Part model, mm, in its own coordinate system. Round coordinates to 2 decimals unless told otherwise and drop trailing zeros. Write each loop counter-clockwise with the first axis right and the second up, starting at its lowest first coordinate (ties: lowest second). Pieces come first, ordered by that corner, then holes. Notation, with made-up numbers: M 2,-32.5 L 9,-32.5 A6 ccw 9,-26.5 Z; hole C 3.25,-0.5 d6. An arc over 180 degrees is marked long. Use one line per item in the form item = value. Start each with the question number.
Item 1: Probe L1, parallel to Z at x = 0, y = -6; L2, parallel to Y at x = -2.5, z = 0.25; L3, parallel to X at y = -9, z = 0.25. List the from-to ranges inside material, lowest first.
Item 2: Cut at C-C, the plane z = -2.75. Give the cut face in (x, y), then the cut area to 3 significant figures.
Item 3: Cut at A-A, the plane y = -8.75. Give the cut face in (x, z), then the cut area to 3 significant figures.
Item 4: Cut at B-B, the plane x = 2.5. Give the cut face in (y, z).
Item 5: Flat gauge pins, fed straight in: pin 1 Ø2 at (y, z) = (-7, -2) entering from -X; pin 2 Ø3 at (x, y) = (0.5, -8.5) entering from +Z; pin 3 Ø1.5 at (x, y) = (1, -1.5) entering from +Z. Where does each tip first touch, or does it go through?
Item 6: Mould opens along X. For faces 1 (the face through (0, -2, -2)), 2 (the face through (-1.4, -6.44, 0.06)), 3 (the face through (0.108, -5.916, -0.488)) say: +X half, -X half, draft (parallel to the pull), parting line (faces both ways), or undercut.
from build123d import *

# Parameters (mm, degrees)
F0_R     = 3.5
F1_DEPTH = 2
F2_R     = 1.4
F3_DEPTH = 10
F4_R     = 0.5
F5_DEPTH = 12.001


# Not quite as in the source:
# - a fillet or chamfer that OpenCascade refuses, or shapes differently, is made with other operations: its cross-section is extruded or revolved along the edge and cut away or added


with BuildPart() as f1:
    # F0 (on Front) → F1 (new body)
    with BuildSketch(Plane.XZ):
        Circle(F0_R)
    extrude(amount=F1_DEPTH)

    # F2 (on face) → F3 (join)
    with BuildSketch(Plane.XZ.offset(2)):
        Circle(F2_R)
    extrude(amount=F3_DEPTH)

    # F4 (on face) → F5 (cut, through all)
    with BuildSketch(Plane(origin=(0, 0, 0), x_dir=(-1, 0, 0), z_dir=(0, 1, 0))):
        Circle(F4_R)
    extrude(amount=-F5_DEPTH, mode=Mode.SUBTRACT)

    # F6: fillet of radius 1 on 1 edges, made by hand

    # F6_s1 → F6_t2 (revolve, cut)
    with BuildSketch(Plane.XY):
        with BuildLine():
            ThreePointArc((1.4, -11.0050125629), (1.1416198487, -11.6758329561), (0.5, -12))
            Line((0.5, -12), (1.4, -12))
            Line((1.4, -12), (1.4, -11.0050125629))
        make_face()
    revolve(axis=Axis((0, -12, 0), (0, -1, 0)), mode=Mode.SUBTRACT)


solid = f1.part
Model answer:
q1.L1 = -1.4 to -0.5, 0.5 to 1.4
q1.L2 = -2 to 0
q1.L3 = -1.38 to -0.43, 0.43 to 1.38
q2.outline = M -2.17,-2 L 2.17,-2 L 2.17,0 L -2.17,0 Z
q2.area = 8.66 mm²
q3.outline = C 0,0 d2.8; hole C 0,0 d1
q3.area = 5.37 mm²
q4.outline = M -2,-2.45 L 0,-2.45 L 0,2.45 L -2,2.45 Z
q5.pin_1 = -0.98
q5.pin_2 = 1.4
q5.pin_3 = 3.49
q6.face_1 = draft
q6.face_2 = parting line
q6.face_3 = undercut
